```python
from build123d import *

# Parameters (mm, degrees)
CYLINDER070_R          = 2.2
CYLINDER070_DEPTH      = 20
CYLINDER069_R          = 2.2
CYLINDER069_DEPTH      = 20
CYLINDER068_R          = 5
CYLINDER068_DEPTH      = 16
CYLINDER065_W          = 8
CYLINDER065_H          = 16
CYLINDER065_ANGLE      = 180
BOX052_W               = 30
BOX052_H               = 5
BOX052_DEPTH           = 16
CUT076_PITCH_ANGLE     = 90
CUT076_PLACEMENT_ANGLE = 90


with BuildPart() as zylinder059:
    # Cylinder070 → Cylinder070 (new body)
    with BuildSketch(Plane(origin=(10, 9, 8), x_dir=(1, 0, 0), z_dir=(0, -1, 0))):
        Circle(CYLINDER070_R)
    extrude(amount=CYLINDER070_DEPTH)


with BuildPart() as zylinder058:
    # Cylinder069 → Cylinder069 (new body)
    with BuildSketch(Plane(origin=(-10, 9, 8), x_dir=(1, 0, 0), z_dir=(0, -1, 0))):
        Circle(CYLINDER069_R)
    extrude(amount=CYLINDER069_DEPTH)


with BuildPart() as zylinder057:
    # Cylinder068 → Cylinder068 (new body)
    with BuildSketch(Plane.XY):
        Circle(CYLINDER068_R)
    extrude(amount=CYLINDER068_DEPTH)


with BuildPart() as zylinder054:
    # Cylinder065 → Cylinder065 (revolve)
    with BuildSketch(Plane(origin=(0, 0, 0), x_dir=(-1, 0, 0), z_dir=(0, 1, 0))):
        with Locations((4, 8)):
            Rectangle(CYLINDER065_W, CYLINDER065_H)
    revolve(axis=Axis((0, 0, 0), (0, 0, 1)), revolution_arc=CYLINDER065_ANGLE)


with BuildPart() as y_mount_top:
    # Box052 → Box052 (new body)
    with BuildSketch(Plane(origin=(-15, -5, 0), x_dir=(1, 0, 0), z_dir=(0, 0, 1))):
        with Locations((15, 2.5)):
            Rectangle(BOX052_W, BOX052_H)
    extrude(amount=BOX052_DEPTH)

    # Fusion035: union Zylinder054
    add(zylinder054.part)

    # Cut072: cut Zylinder057
    add(zylinder057.part, mode=Mode.SUBTRACT)

    # Cut075: cut Zylinder058
    add(zylinder058.part, mode=Mode.SUBTRACT)

    # Cut076: cut Zylinder059
    add(zylinder059.part, mode=Mode.SUBTRACT)


with BuildPart() as y_mount_top_1:
    # Cut076 pitch: moved
    add(y_mount_top.part.rotate(Axis((0, 0, 0), (0, 1, 0)), CUT076_PITCH_ANGLE))


with BuildPart() as y_mount_top_2:
    # Cut076 placement: moved
    add(y_mount_top_1.part.moved(Location((-9.75, -14.15, 29.85))).rotate(Axis((-9.75, -14.15, 29.85), (0, 0, 1)), CUT076_PLACEMENT_ANGLE))


solid = y_mount_top_2.part
```
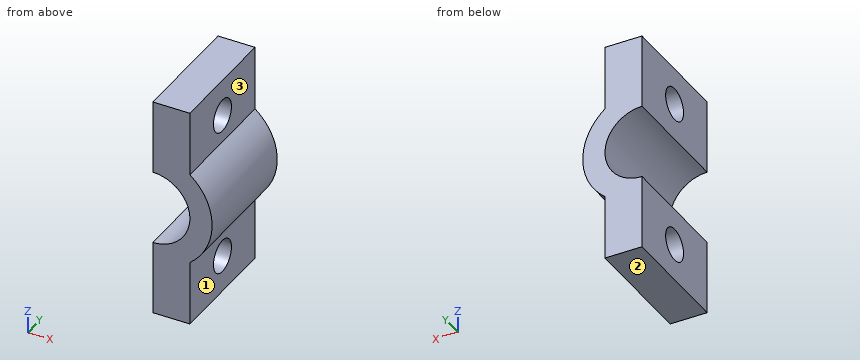
The listing builds one solid part. Answer for the finished solid, in the listing's coordinates (mm). Face numbers are marked on the shaded views. A direction names the side the tool comes from. Coordinates: 2 decimals unless noted, no trailing zeros. Loops run counter-clockwise (first coordinate to the right, second up) from the corner with the lowest first, then second, coordinate; pieces in that order, holes last. Notation, with made-up numbers: (-2, 42) - (40, 42) arc R23 ccw to (40, 80) - close; hole circle Ø5 at (-27, 70.5). An arc over 180 degrees is marked (long way). Write item = value, one per line.
1) Section C-C (y = -6.15) is taken. Determine the outline of the cut face in (x, z) (3 decimals).
Responses:
outline = (-9.75, 14.85) - (-4.75, 14.85) - (-4.75, 17.65) - (-9.75, 17.65) - close; (-9.75, 22.05) - (-4.75, 22.05) - (-4.75, 23.605) arc R8 ccw to (-4.75, 36.095) - (-4.75, 37.65) - (-9.75, 37.65) - (-9.75, 34.85) arc R5 cw to (-9.75, 24.85) - close; (-9.75, 42.05) - (-4.75, 42.05) - (-4.75, 44.85) - (-9.75, 44.85) - close
2) Section D-D (y = -3) is taken. Determine the outline of the cut face in (x, z) (3 decimals).
Responses:
outline = (-9.75, 14.85) - (-4.75, 14.85) - (-4.75, 23.605) arc R8 ccw to (-4.75, 36.095) - (-4.75, 44.85) - (-9.75, 44.85) - (-9.75, 34.85) arc R5 cw to (-9.75, 24.85) - close
3) Which of the six approach directions +Z, -Z, +X, -X, +Y, -Y give full straight-line access (tool end or side, diameter ignored) to the marked faces 1, 2 and 3?
Responses:
face_1 = -Z, +X, +Y, -Y
face_2 = -Z, +X, -X, +Y, -Y
face_3 = +Z, +X, +Y, -Y
4) Section B-B (x = -5.25) is taken. Determine the outline of the cut face in (y, z), plus the area to 3 significant figures.
Responses:
outline = (-14.15, 14.85) - (1.85, 14.85) - (1.85, 27.67) - (-14.15, 27.67) - close; (-14.15, 32.03) - (1.85, 32.03) - (1.85, 44.85) - (-14.15, 44.85) - close; hole circle Ø4.4 at (-6.15, 19.85); hole circle Ø4.4 at (-6.15, 39.85)
area = 380 mm^2
5) Section A-A (z = 19.85) is taken. Determine the outline of the cut face in (x, y).
Responses:
outline = (-9.75, -14.15) - (-4.75, -14.15) - (-4.75, -8.35) - (-9.75, -8.35) - close; (-9.75, -3.95) - (-4.75, -3.95) - (-4.75, 1.85) - (-9.75, 1.85) - close
6) Each of these flat-tipped pins is pushed along its axis until it touches: P1, Ø9.5, axis at y = -5.5, z = 18, coming from the +X side; P2, Ø3, axis at y = -6.5, z = 34, coming from the -X side; P3, Ø4, axis at y = -6.15, z = 39.85, coming from the +X side; P4, Ø9.5, axis at y = -6.5, z = 40, coming from the +X side. Where does it stop, or does it pass through?
Responses:
P1 = -4.75
P2 = -9.75
P3 = through
P4 = -3.85
7) Find the intervals of material crossed by line 1 along Y through (x, z) = (-8, 39.85); line 2 along Z through (x, y) = (-6, -6.15); line 3 along Z through (x, y) = (-6.8, -6.15), in increasing order.
Responses:
line_1 = -14.15 to -8.35, -3.95 to 1.85
line_2 = 14.85 to 17.65, 22.05 to 26.54, 33.16 to 37.65, 42.05 to 44.85
line_3 = 14.85 to 17.65, 22.05 to 25.81, 33.89 to 37.65, 42.05 to 44.85
